from build123d import *

# Parameters (mm, degrees)
F0_R     = 2.5
F1_DEPTH = 3


with BuildPart() as f1:
    # F0 (on Top) → F1 (new body)
    with BuildSketch(Plane.XY):
        Polygon((0, 8), (0, 0), (41, 0), (41, 26), (67, 26), (67, 0), (80, 0), (80, 40), (32, 40), (32, 8), align=None)
        with Locations((4, 4)):
            Circle(F0_R, mode=Mode.SUBTRACT)
        with Locations((76, 4)):
            Circle(F0_R, mode=Mode.SUBTRACT)
        with Locations((76, 36)):
            Circle(F0_R, mode=Mode.SUBTRACT)
    extrude(amount=F1_DEPTH)


solid = f1.part
Read the model definition and answer for the solid it produces. Units are mm, in the model's axes. A direction names the side the tool comes from. Round coordinates to 2 decimals unless told otherwise and drop trailing zeros. Loops run counter-clockwise (first coordinate to the right, second up) from the corner with the lowest first, then second, coordinate; pieces in that order, holes last. Notation, with made-up numbers: (-17.75, 84.5) - (24.25, 84.5) arc R24 ccw to (24.25, 104.5) - close; hole circle Ø7 at (86.25, -21.75). An arc over 180 degrees is marked (long way). One line per question, with ' | ' between items. Start each with the question number.
Q1. Section A-A on y = 4 is taken. Give the vertices of the cut face in (x, z), plus the area to 3 significant figures.
Q2. For faces 1 (the flat face through (0, 4, 1)), 2 (the flat face through (67, 13, 1)), 3 (the flat face through (32, 24, 1)), determine the directions among +Z, -Z, +X, -X, +Y, -Y from which every point of the face is accessible in a straight line to the end or side of a thin tool.
Q3. Find the intervals of material crossed by L1, parallel to Y at x = 76, z = 1.15; L2, parallel to X at y = 2, z = 1.9; L3, parallel to X at y = 7, z = 2.8, in increasing order.
Q4. Section C-C on y = 24.5 is taken. Give the vertices of the cut face in (x, z).
Q5. Section B-B on x = 4 is taken. Give the vertices of the cut face in (y, z).
Q6. Section D-D on x = 76 is taken. Give the vertices of the cut face in (y, z).
Q7. For a pull along Y with two mould halves and no side action, classify faces 4 (the flat face through (16, 8, 1)), 5 (the cylindrical face through (74, 34.5, 1.5)), 6 (the flat face through (20, 0, 1)) as +Y half, -Y half, draft (parallel to the pull), parting line (faces both ways), or undercut.
Q8. Flat-ended cylindrical pins translate along their axes: pin 1 (0.9 mm diameter, centred on y = 15, z = 2, fed in from -X); pin 2 (4.5 mm diameter, centred on x = 4, y = 4, fed in from +Z); pin 3 (0.9 mm diameter, centred on x = 14, z = 1.5, fed in from +Y). Find the tip coordinate at first contact, or state that the pin passes through.
Established:
1) outline: (0, 0) - (1.5, 0) - (1.5, 3) - (0, 3) - close; (6.5, 0) - (41, 0) - (41, 3) - (6.5, 3) - close; (67, 0) - (73.5, 0) - (73.5, 3) - (67, 3) - close; (78.5, 0) - (80, 0) - (80, 3) - (78.5, 3) - close | area: 132 mm²
2) face 1: +Z, -Z, -X, +Y, -Y | face 2: +Z, -Z, -Y | face 3: +Z, -Z, -X, +Y
3) L1: 0 to 1.5, 6.5 to 33.5, 38.5 to 40 | L2: 0 to 2.5, 5.5 to 41, 67 to 74.5, 77.5 to 80 | L3: 0 to 41, 67 to 80
4) outline: (32, 0) - (41, 0) - (41, 3) - (32, 3) - close; (67, 0) - (80, 0) - (80, 3) - (67, 3) - close
5) outline: (0, 0) - (1.5, 0) - (1.5, 3) - (0, 3) - close; (6.5, 0) - (8, 0) - (8, 3) - (6.5, 3) - close
6) outline: (0, 0) - (1.5, 0) - (1.5, 3) - (0, 3) - close; (6.5, 0) - (33.5, 0) - (33.5, 3) - (6.5, 3) - close; (38.5, 0) - (40, 0) - (40, 3) - (38.5, 3) - close
7) face 4: +Y half | face 5: undercut | face 6: -Y half
8) pin 1: x = 32 | pin 2: through | pin 3: y = 8
